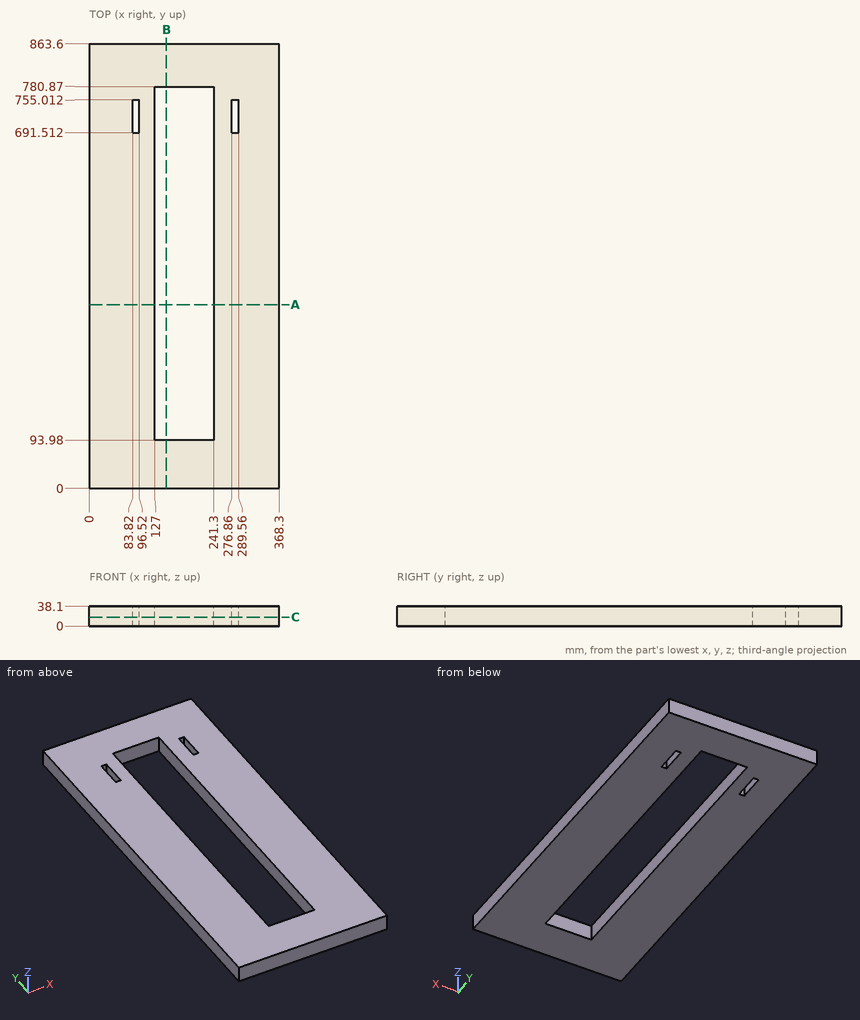
Part print with two shaded views. Sizes in mm from the minimum x, y, z corner. Round coordinates to 2 decimals unless told otherwise and drop trailing zeros. Order: outer loops, then holes, each group sorted by start corner. A loop starts at its lowest first (then second) coordinate and runs counter-clockwise, first axis right, second up. Notation, with made-up numbers: M 45.5,43 L 67.5,43 A28 cw 67.5,76 Z; hole C -37.5,1 d7. An arc over 180 degrees is marked long. Answer in a Markdown table with one row per item. Add a question column.
Q1. Cut at B-B on x = 149.5. Give the cut face in (y, z), and give its area (3 significant figures).
Q2. Cut at A-A on y = 357. Give the cut face in (x, z), and give its area (3 significant figures).
Q3. Wall check: L1, parallel to X at y = 705, z = 32; L2, parallel to Y at x = 200.5, z = 34.5; L3, parallel to X at y = 274, z = 31. Give the ranges that are in metal, low to high. Write a range as from..to.
Q4. Pin check, flat tip, straight feed: pin 1 (6 mm diameter, centred on x = 288.5, y = 229, fed in from -Z). Stop position of the tip, or through.
Q5. Cut at C-C on z = 17.5. Give the cut face in (x, y).
Established:
| question | item | result |
|---|---|---|
| 1 | outline | M 0,0 L 93.98,0 L 93.98,38.1 L 0,38.1 Z; M 780.87,0 L 863.6,0 L 863.6,38.1 L 780.87,38.1 Z |
| 1 | area | 6,730 mm2 |
| 2 | outline | M 0,0 L 127,0 L 127,38.1 L 0,38.1 Z; M 241.3,0 L 368.3,0 L 368.3,38.1 L 241.3,38.1 Z |
| 2 | area | 9,680 mm2 |
| 3 | L1 | x = 0..83.82, 96.52..127, 241.3..276.86, 289.56..368.3 |
| 3 | L2 | y = 0..93.98, 780.87..863.6 |
| 3 | L3 | x = 0..127, 241.3..368.3 |
| 4 | pin 1 | stops at z = 0 |
| 5 | outline | M 0,0 L 368.3,0 L 368.3,863.6 L 0,863.6 Z; hole M 83.82,691.51 L 96.52,691.51 L 96.52,755.01 L 83.82,755.01 Z; hole M 127,93.98 L 241.3,93.98 L 241.3,780.87 L 127,780.87 Z; hole M 276.86,691.51 L 289.56,691.51 L 289.56,755.01 L 276.86,755.01 Z |
